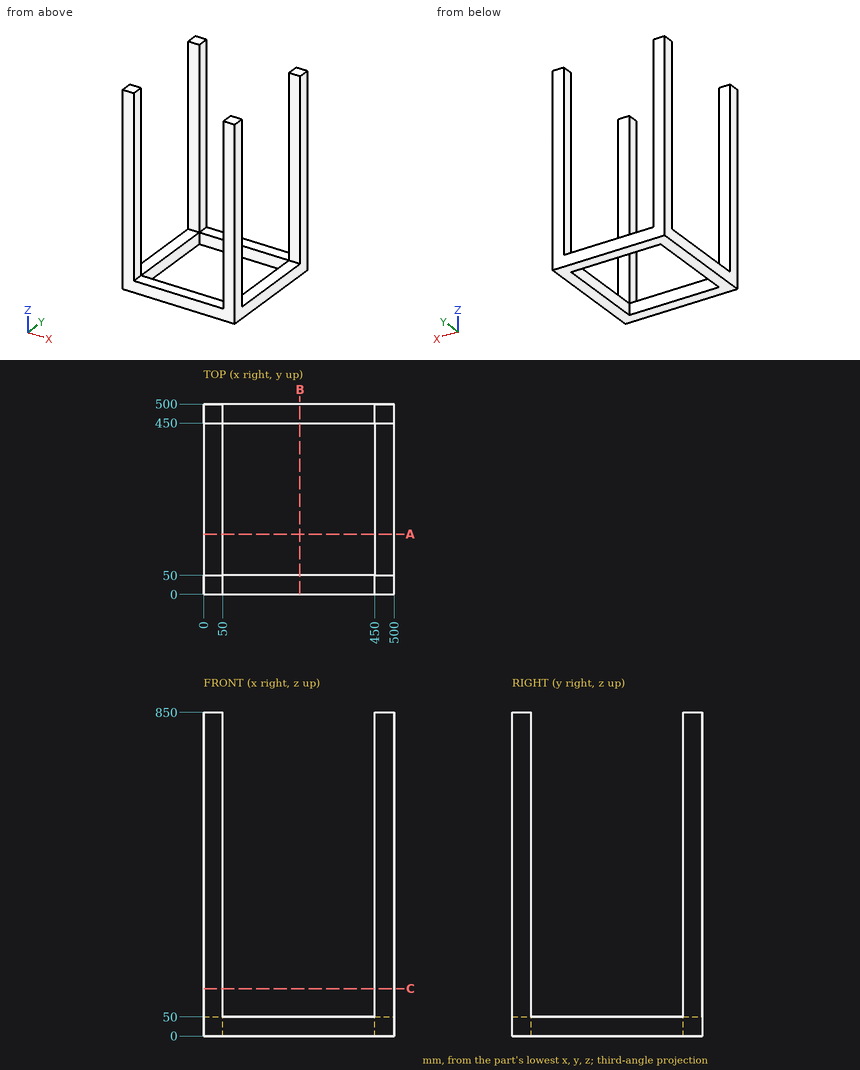
Can you work these out from the drawing? Everything is in mm from the part's minimum corner. Round coordinates to 2 decimals unless told otherwise and drop trailing zeros. Loops run counter-clockwise (first coordinate to the right, second up) from the corner with the lowest first, then second, coordinate; pieces in that order, holes last. Notation, with made-up numbers: (46, -36.5) -> (59, -36.5) arc R16 cw to (59, -17.5) -> close; hole circle Ø3 at (-17.75, 60). An arc over 180 degrees is marked (long way). One line per question, with ' | ' between items.
(1) If we section it at A-A on y = 158.5: List the corners of the cut face in (x, z) for me, and give its area (3 significant figures).
Model answer:
outline: (0, 0) -> (50, 0) -> (50, 50) -> (0, 50) -> close; (450, 0) -> (500, 0) -> (500, 50) -> (450, 50) -> close | area: 5,000 mm^2
(2) If I drill on probe 1 along Y at (x, z) = (463, 241.5); probe 2 along Z at (x, y) = (29, 180), over which ranges is the centre line in solid material (lowest first)?
Model answer:
probe 1: y = 0 to 50, 450 to 500 | probe 2: z = 0 to 50
(3) For pin 1 Ø15 at (x, y) = (273.5, 465) entering from +Z, with a flat end and sliding along its axis, tell me the tip position at first contact or that it passes through.
Model answer:
pin 1: stops at z = 50
(4) If we section it at C-C on z = 124.5: List the corners of the cut face in (x, y) for me.
Model answer:
outline: (0, 0) -> (50, 0) -> (50, 50) -> (0, 50) -> close; (0, 450) -> (50, 450) -> (50, 500) -> (0, 500) -> close; (450, 0) -> (500, 0) -> (500, 50) -> (450, 50) -> close; (450, 450) -> (500, 450) -> (500, 500) -> (450, 500) -> close
